Geometry: final body of the model. Coordinates: model frame, mm. Face numbers are marked on the shaded views. A direction names the side the tool comes from. Give positions to 0.01 mm unless a question says otherwise; leave off trailing zeros. Write each loop counter-clockwise with the first axis right and the second up, starting at its lowest first coordinate (ties: lowest second). Pieces come first, ordered by that corner, then holes. Notation, with made-up numbers: M -27,59.25 L -14,59.25 A16 cw -14,77.25 Z; hole C 66,88.5 d8. An arc over 180 degrees is marked long. Use one line per item in the form item = value. Start each with the question number.
Item 1: Contact query for a flat-ended pin moving along its axis: P1, Ø5, axis at x = 34, y = 8.5, coming from the +Z side. Output: stop coordinate, or through.
Item 2: Section query A-A on y = 8.25. Return loops of the section in (x, z).
Item 3: Section query B-B on x = 82. Return loops of the section in (y, z).
Item 4: Section query C-C on z = 3. Return loops of the section in (x, y).
Item 5: Material intervals for line 1 along Z through (x, y) = (70.5, 10); line 2 along Z through (x, y) = (5.5, 5.25); line 3 along X through (y, z) = (9, 6.5), sorted ascending. Write a range as from..to.
Item 6: Access query for the marked faces 1 and 2. Directions: +Z, -Z, +X, -X, +Y, -Y. A direction counts if a zero-diameter tool reaches every point of the face in a straight line with its end or side. Return the directions, or none.
from build123d import *

# Parameters (mm, degrees)
F1_DEPTH = 12


# Not quite as in the source:
# - a feature names something its author has since deleted; it is built from what else it names


with BuildPart() as f1:
    # F0 (on Front) → F1 (new body)
    with BuildSketch(Plane.XZ):
        Polygon((7.9674337148, 13.8), (0, 0), (89, 0), (89, 12), (9.0066641994, 12), align=None)
    extrude(amount=-F1_DEPTH)


solid = f1.part
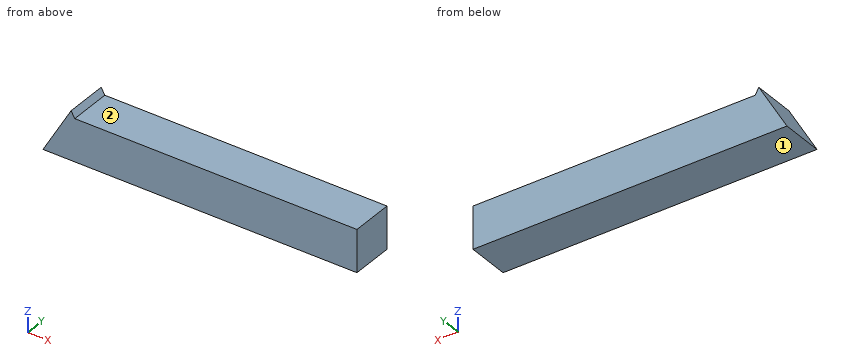
Answer sheet:
q1.P1 = 12
q2.outline = M 0,0 L 89,0 L 89,12 L 9.01,12 L 7.97,13.8 Z
q3.outline = M 0,0 L 12,0 L 12,12 L 0,12 Z
q4.outline = M 1.73,0 L 89,0 L 89,12 L 1.73,12 Z
q5.line_1 = 0..12
q5.line_2 = 0..9.53
q5.line_3 = 3.75..89
q6.face_1 = -Z, +X, -X, +Y, -Y
q6.face_2 = +Z, +X, +Y, -Y
